Read the model definition and answer for the solid it produces. Units are mm, in the model's axes. Face numbers are marked on the shaded views. A direction names the side the tool comes from. Coordinates: 2 decimals unless noted, no trailing zeros. Write each loop counter-clockwise with the first axis right and the second up, starting at its lowest first coordinate (ties: lowest second). Pieces come first, ordered by that corner, then holes. Notation, with made-up numbers: (-13, -29.5) -> (35, -29.5) arc R27 ccw to (35, -8.5) -> close; hole circle Ø1 at (5.25, -25). An arc over 180 degrees is marked (long way). Answer as a JSON object with one key per item and string values. Group by question number.
(1) Find section B-B (x = -19). Give the vertices of the cut face in (y, z), then the cut area to 3 significant figures.
(2) Find section A-A (z = -4.5). Give the vertices of the cut face in (x, y).
(3) Which of the six approach directions +Z, -Z, +X, -X, +Y, -Y give full straight-line access (tool end or side, diameter ignored) to the marked faces 4 and 5?
(4) Find section D-D (y = -19). Give the vertices of the cut face in (x, z).
(5) Straight lines are drawn through the part: L1, parallel to Y at x = -15, z = -22; L2, parallel to X at y = -17, z = -23; L3, parallel to Z at x = 5, y = -36. For each, find the intervals that lie inside material, in ascending order.
(6) Find section C-C (y = -5.5). Give the vertices of the cut face in (x, z).
(7) Flat-ended cylindrical pins translate along their axes: P1, Ø3, axis at x = 15, y = -17.5, coming from the +Z side; P2, Ø8.5, axis at x = 15, y = -42.5, coming from the +Z side; P3, Ø7, axis at x = 13.44, z = -13.44, coming from the +Y side. Find the tip coordinate at first contact, or state that the pin passes through.
(8) For a pull along Z with two mould halves and no side action, classify the marked faces 1, 2 and 3 as +Z half, -Z half, draft (parallel to the pull), parting line (faces both ways), or undercut.
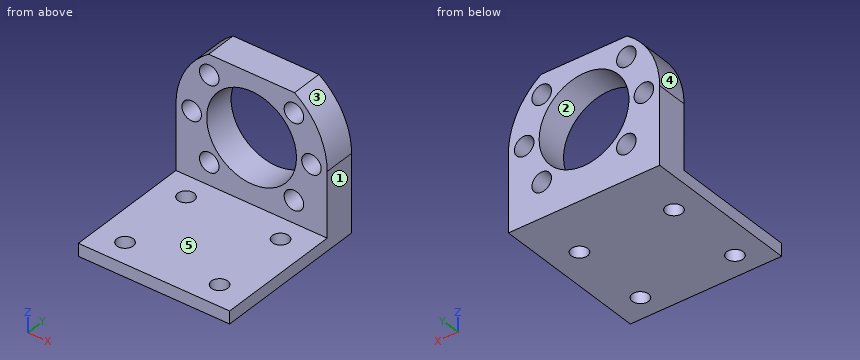
from build123d import *

# Parameters (mm, degrees)
F0_R     = 3.1
F0_R_2   = 14.25
F1_DEPTH = 10
F2_W     = 48
F2_H     = 4
F3_DEPTH = 40
F4_R     = 2.6
F5_DEPTH = 4


with BuildPart() as f1:
    # F0 (on Front) → F1 (new body)
    with BuildSketch(Plane.XZ):
        with BuildLine():
            Line((13.63589, 19.75), (-13.63589, 19.75))
            ThreePointArc((-13.63589, 19.75), (-21.251604, 11.152099), (-24, 0))
            Line((-24, 0), (-24, -24.5))
            Line((-24, -24.5), (24, -24.5))
            Line((24, -24.5), (24, 0))
            ThreePointArc((24, 0), (21.251604, 11.152099), (13.63589, 19.75))
        make_face()
        with Locations((-13.435029, -13.435029)):
            Circle(F0_R, mode=Mode.SUBTRACT)
        with Locations((13.435029, -13.435029)):
            Circle(F0_R, mode=Mode.SUBTRACT)
        with Locations((-19, 0)):
            Circle(F0_R, mode=Mode.SUBTRACT)
        with Locations((-13.435029, 13.435029)):
            Circle(F0_R, mode=Mode.SUBTRACT)
        Circle(F0_R_2, mode=Mode.SUBTRACT)
        with Locations((19, 0)):
            Circle(F0_R, mode=Mode.SUBTRACT)
        with Locations((13.435029, 13.435029)):
            Circle(F0_R, mode=Mode.SUBTRACT)
    extrude(amount=F1_DEPTH)

    # F2 (on face) → F3 (join)
    with BuildSketch(Plane.XZ.offset(10)):
        with Locations((0, -22.5)):
            Rectangle(F2_W, F2_H)
    extrude(amount=F3_DEPTH)

    # F4 (on face) → F5 (cut, through all)
    with BuildSketch(Plane.XY.offset(-20.5)):
        with Locations((-15, -17.5)):
            Circle(F4_R)
        with Locations((-15, -42.5)):
            Circle(F4_R)
        with Locations((15, -42.5)):
            Circle(F4_R)
        with Locations((15, -17.5)):
            Circle(F4_R)
    extrude(amount=-F5_DEPTH, mode=Mode.SUBTRACT)


solid = f1.part
Results below:
{
 "1": {"outline": "(-50, -24.5) -> (0, -24.5) -> (0, -3.1) -> (-10, -3.1) -> (-10, -20.5) -> (-50, -20.5) -> close; (-10, 3.1) -> (0, 3.1) -> (0, 14.66) -> (-10, 14.66) -> close", "area": "490 mm2"},
 "2": {"outline": "(-24, -10) -> (-13.52, -10) -> (-13.52, 0) -> (-24, 0) -> close; (13.52, -10) -> (24, -10) -> (24, 0) -> (13.52, 0) -> close"},
 "3": {"face 4": "+Z, -X, +Y, -Y", "face 5": "+Z, +X, -X, -Y"},
 "4": {"outline": "(-24, -24.5) -> (-17.12, -24.5) -> (-17.12, -20.5) -> (-24, -20.5) -> close; (-12.88, -24.5) -> (12.88, -24.5) -> (12.88, -20.5) -> (-12.88, -20.5) -> close; (17.12, -24.5) -> (24, -24.5) -> (24, -20.5) -> (17.12, -20.5) -> close"},
 "5": {"L1": "y = -50 to -45.1, -39.9 to -20.1, -14.9 to 0", "L2": "x = -24 to -17.55, -12.45 to 12.45, 17.55 to 24", "L3": "z = -24.5 to -20.5"},
 "6": {"outline": "(-24, -24.5) -> (24, -24.5) -> (24, 0) arc R24 ccw to (13.64, 19.75) -> (-13.64, 19.75) arc R24 ccw to (-24, 0) -> close; hole circle Ø6.2 at (-19, 0); hole circle Ø6.2 at (-13.44, -13.44); hole circle Ø6.2 at (-13.44, 13.44); hole circle Ø28.5 at (0, 0); hole circle Ø6.2 at (13.44, -13.44); hole circle Ø6.2 at (13.44, 13.44); hole circle Ø6.2 at (19, 0)"},
 "7": {"P1": "passes through", "P2": "stops at z = -20.5", "P3": "stops at y = 0"},
 "8": {"face 1": "draft", "face 2": "undercut", "face 3": "+Z half"}
}
